Autodesk Inventor part; units mm, degrees
ref_plane "YZ Plane" through (0, 0, 0) normal (1, 0, 0) x (0, 1, 0)
ref_plane "XZ Plane" through (0, 0, 0) normal (0, 1, 0) x (-1, 0, 0)
ref_plane "XY Plane" through (0, 0, 0) normal (0, 0, 1) x (1, 0, 0)
sketch "Sketch1" plane through (0, 0, 0) normal (1, 0, 0) x (0, 1, 0)
  line L0 (10, 24) -> (0, 24)
  line L1 (0, 24) -> (0, 0)
  line L2 (0, 0) -> (10, 0)
  line L3 (10, 0) -> (10, 24)
  line L4 (10, 24) -> (0, 24)
  line L5 (0, 24) -> (0, 12)
  line L6 (0, 12) -> (10, 12)
  line L7 (10, 12) -> (10, 24)
  dimension "d0" = 24
  dimension "d1" = 10
  dimension "d2" = 12
extrude "Extrusion1" add sketch "Sketch1" along normal blind 19 contours L3 L6 L1 L0
extrude "Extrusion2" add sketch "Sketch1" along normal blind 9 contours L3 L2 L1 L6
sketch "Sketch2" plane through (9, 0, 0) normal (1, 0, 0) x (0, 0, -1)
  circle A0 centre (-6, 5) radius 2
  line L0 (0, 10) -> (-12, 10)
  line L1 (0, 0) -> (0, 10)
  circle A1 centre (-6, 5) radius 1.5
  line L2 (-7.2, 5.9) -> (-4.8, 5.9)
  dimension "d7" = 4
  dimension "d8" = 5
  dimension "d9" = 6
  dimension "d10" = 3
  dimension "d11" = 2.4
extrude "Extrusion3" add sketch "Sketch2" along normal blind 1
extrude "Extrusion4" add sketch "Sketch2" along normal blind 10 contours A1 L2 picked at (-5.5775, 4.8311)
extrude "Extrusion5" add sketch "Sketch2" along normal blind 1 contours L2 A1 picked at (-5.6796, 5.9839)
sketch "Sketch3" plane through (19, 0, 0) normal (1, 0, 0) x (0, 0, -1)
  line L0 (-24, 10) -> (-24, 0)
  line L1 (-24, 10) -> (-12, 10)
  line L2 (-12, 10) -> (-12, 0)
  line L3 (-12, 0) -> (-24, 0)
  line L4 (-24, 0) -> (-24, 10)
  line L5 (-12, 10) -> (-24, 10)
  line L6 (-24, 0) -> (-12, 0)
  line L7 (-21.5, 10) -> (-14.5, 10)
  line L8 (-14.5, 10) -> (-14.5, 0)
  line L9 (-14.5, 0) -> (-21.5, 0)
  line L10 (-21.5, 0) -> (-21.5, 10)
  arc A0 (-21.5, 10) -> (-21.5, 0) centre (-17.75, 5) ccw
  arc A1 (-14.5, 0) -> (-14.5, 10) centre (-18.25, 5) ccw
  point P0 (0, 0)
  dimension "d18" = 2.5
  dimension "d19" = 2.5
  dimension "d20" = 7
extrude "Extrusion6" cut sketch "Sketch3" against normal blind 15 contours L1 A0 L0 | A0 L3 L0
extrude "Extrusion7" cut sketch "Sketch3" against normal blind 15 contours L1 L2 A1 | A1 L2 L3
extrude "Extrusion8" add sketch "Sketch3" along normal blind 4 contours A0 L10 | L1 L8 L3 L10 | A1 L8
sketch "Sketch4" plane through (23, 0, 0) normal (1, 0, 0) x (0, 0, -1)
  line L0 (-12, 5) -> (-12, 0)
  line L1 (-23.9948, 0) -> (-12, 0)
  line L2 (-12, 0) -> (-12, 5)
  line L3 (-12, 5) -> (-23.9948, 5)
  line L4 (-23.9948, 5) -> (-23.9948, 0)
  point P0 (0, 0)
extrude "Extrusion9" cut sketch "Sketch4" against normal blind 4
sketch "Sketch5" plane through (23, 0, 0) normal (1, 0, 0) x (0, 0, -1)
  point P0 (0, 0)
sketch "Sketch6" plane through (0, 10, 0) normal (0, 1, 0) x (1, 0, 0)
  line L0 (23, -23.9948) -> (23, -12)
  line L1 (19, -12) -> (19, -14.5)
  line L2 (23, -21.4808) -> (19, -21.4808)
  line L3 (19, -21.4808) -> (19, -14.5)
  line L4 (19, -14.5) -> (23, -14.5)
  line L5 (23, -14.5) -> (23, -21.4808)
  point P0 (0, 0)
extrude "Extrusion10" cut sketch "Sketch6" against normal blind 8
equation "\"d19\" = d18"
properties part number "motorcek"
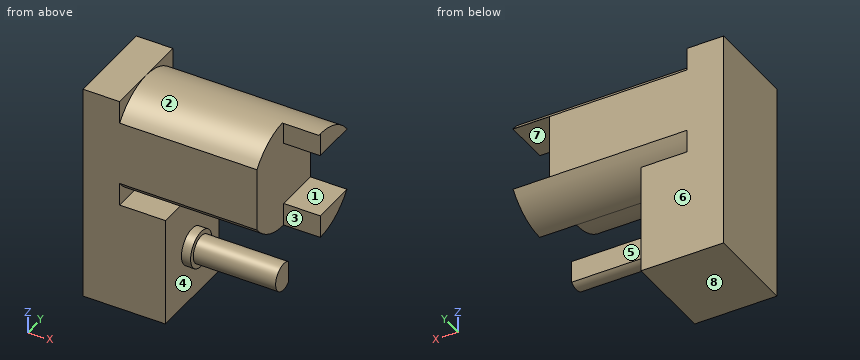
Read the model definition and answer for the solid it produces. Units are mm, in the model's axes. Face numbers are marked on the shaded views. A direction names the side the tool comes from. Give positions to 0.01 mm unless a question says otherwise; leave off trailing zeros. Write each loop counter-clockwise with the first axis right and the second up, starting at its lowest first coordinate (ties: lowest second). Pieces come first, ordered by that corner, then holes. Notation, with made-up numbers: (-35.5, -18) - (-9.5, -18) arc R18 cw to (-9.5, 11) - close; hole circle Ø6 at (23.25, 16). An arc over 180 degrees is marked (long way). Answer in a Markdown table with one row per item. Add a question column.
Item 1: Section C-C, the plane y = 4.25 is taken. Write down the section's boundary in (x, z), and give its area (3 significant figures).
Item 2: Section A-A, the plane x = 9.5 is taken. Write down the section's boundary in (y, z), and give its area (3 significant figures).
Item 3: Determine the mould class of the marked faces 6, 7 and 8 for opening direction Z: pulls with the +Z half, pulls with the -Z half, needs draft (parallel to the pull), parting line crosses it, or undercut.
Item 4: Flat-ended cylindrical pins translate along their axes: P1, Ø0.7, axis at x = 15.5, z = 6, coming from the +Y side; P2, Ø5, axis at y = 6.5, z = 8, coming from the +X side; P3, Ø0.8, axis at x = 20.5, z = 22.5, coming from the -Y side. Find the tip coordinate at first contact, or state that the pin passes through.
Item 5: Section D-D, the plane x = 16.25 is taken. Write down the section's boundary in (y, z).
Item 6: A tool of negligible diameter and unlimited length cuts with its end or side. For the marked faces 1, 2, 3, 4 and 5, from which of +Z, -Z, +X, -X, +Y, -Y can it reach the whole face along a straight path? Write none if from no direction.
Item 7: Section B-B, the plane z = 6 is taken. Write down the section's boundary in (x, y).
Item 8: Find the intervals of material crossed by L1, parallel to X at y = 2.75, z = 16.25; L2, parallel to X at y = 2.5, z = 4; L3, parallel to Y at x = 15.5, z = 6, in increasing order.
Recorded:
| question | item | result |
|---|---|---|
| 1 | outline | (0, 0) - (9, 0) - (9, 4.15) - (10, 4.15) - (10, 4.7) - (19, 4.7) - (19, 7.3) - (10, 7.3) - (10, 7.85) - (9, 7.85) - (9, 12) - (4, 12) - (4, 12.05) - (19, 12.05) - (19, 23.95) - (4, 23.95) - (4, 24) - (0, 24) - close |
| 1 | area | 362 mm2 |
| 2 | outline | (0, 14.5) arc R6.25 ccw to (10, 14.5) - (10, 21.5) arc R6.25 ccw to (0, 21.5) - close; circle Ø4 at (5, 6) |
| 2 | area | 118 mm2 |
| 3 | face 6 | needs draft |
| 3 | face 7 | undercut |
| 3 | face 8 | pulls with the -Z half |
| 4 | P1 | stops at y = 5.9 |
| 4 | P2 | stops at x = 19 |
| 4 | P3 | stops at y = 5 |
| 5 | outline | (0, 14.5) arc R6.25 ccw to (10, 14.5) - (10, 21.5) arc R6.25 ccw to (0, 21.5) - close; (5.9, 4.8) - (5.9, 7.2) arc R1.5 ccw (long way) to start |
| 6 | face 1 | +X, +Y, -Y |
| 6 | face 2 | +Z, +X |
| 6 | face 3 | -Z, +X, -Y |
| 6 | face 4 | +X |
| 6 | face 5 | -Z, +X, +Y |
| 7 | outline | (0, 0) - (9, 0) - (9, 3) - (10, 3) - (10, 3.5) - (19, 3.5) - (19, 5.9) - (10, 5.9) - (10, 7) - (9, 7) - (9, 10) - (0, 10) - close |
| 8 | L1 | x = 0 to 19 |
| 8 | L2 | x = 0 to 9 |
| 8 | L3 | y = 3.5 to 5.9 |
